Geometry: see drawing. Coordinates: mm, zero at the bounding-box minimum. Give positions to 0.01 mm unless a question says otherwise; leave off trailing zeros. Write each loop counter-clockwise with the first axis right and the second up, starting at its lowest first coordinate (ties: lowest second). Pieces come first, ordered by that corner, then holes. Notation, with made-up numbers: M 10.5,-39 L 34.5,-39 A26 ccw 34.5,-18 Z; hole C -24.75,-2 d10. An arc over 180 degrees is marked long. Use one line per item in the form item = value. Start each with the question number.
Item 1: Pull-direction query (X, two-part tool) for the marked faces 1, 2, 3 and 4; classes: released by +X, released by -X, zero draft, split by the parting line, or undercut.
Item 2: Contact query for flat-ended pins moving along their axis: P1, Ø8, axis at x = 11.5, y = 2.5, coming from the +Z side (1 decimal); P2, Ø5, axis at y = 17, z = 39, coming from the +X side (1 decimal); P3, Ø6, axis at y = 13.5, z = 6.5, coming from the +X side (1 decimal). Output: stop coordinate, or through.
Item 3: Section query A-A on z = 31.5. Return loops of the section in (x, y) (1 decimal).
Item 4: Section query D-D on z = 44. Return loops of the section in (x, y).
Item 5: Section query B-B on x = 28. Return loops of the section in (y, z) (1 decimal).
Item 6: Material intervals for line 1 along Z through (x, y) = (24, 12) (1 decimal); line 2 along X through (y, z) = (9.75, 31) (1 decimal); line 3 along X through (y, z) = (9, 30), sorted ascending. Write a range as from..to.
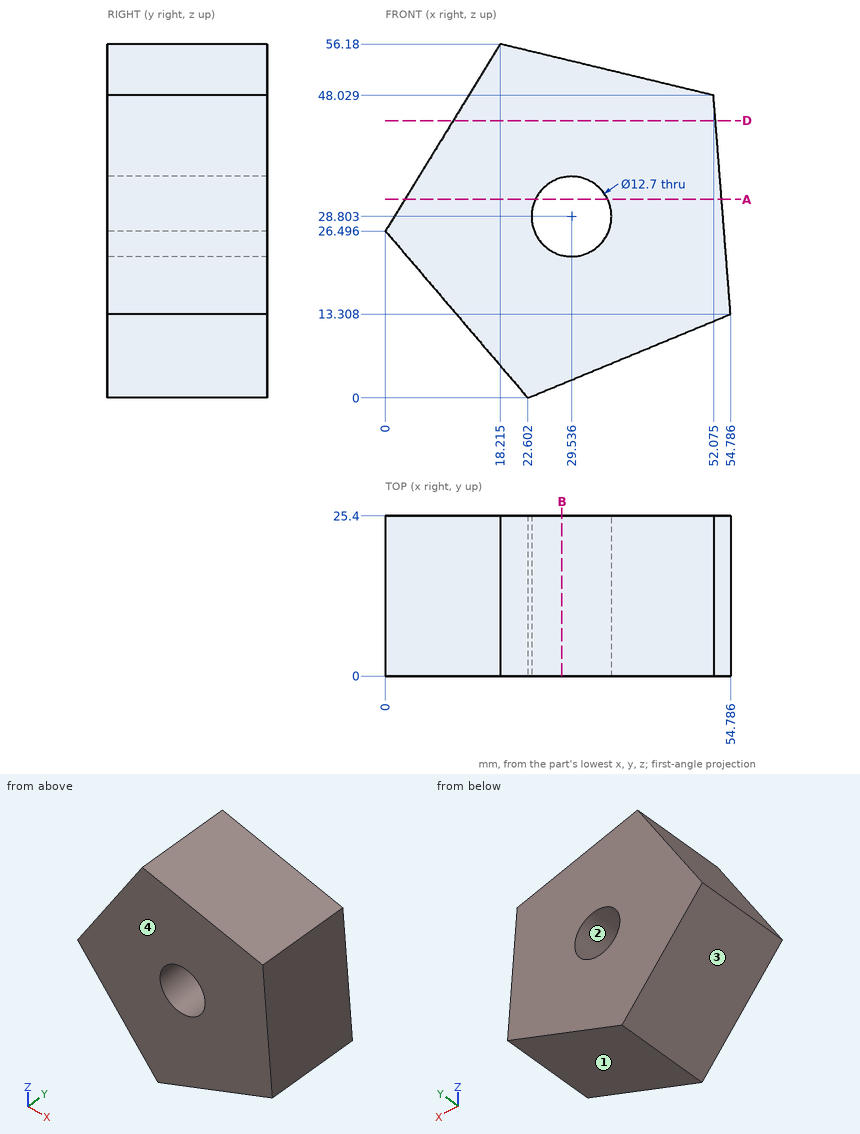
Answer sheet:
q1.face_1 = released by +X
q1.face_2 = undercut
q1.face_3 = released by -X
q1.face_4 = zero draft
q2.P1 = 51.8
q2.P2 = 53
q2.P3 = 45.6
q3.outline = M 3.1,0 L 23.8,0 L 23.8,25.4 L 3.1,25.4 Z; M 35.3,0 L 53.4,0 L 53.4,25.4 L 35.3,25.4 Z
q4.outline = M 10.74,0 L 52.39,0 L 52.39,25.4 L 10.74,25.4 Z
q5.outline = M 0,2.2 L 25.4,2.2 L 25.4,22.6 L 0,22.6 Z; M 0,35 L 25.4,35 L 25.4,53.8 L 0,53.8 Z
q6.line_1 = 0.6..25.7, 31.9..54.8
q6.line_2 = 2.8..23.6, 35.5..53.4
q6.line_3 = 2.15..23.3, 35.77..53.48
